Here's how the part is built. I have some questions about the finished solid (model axes, mm). Face numbers are marked on the shaded views. A direction names the side the tool comes from. Coordinates: 2 decimals unless noted, no trailing zeros. Loops run counter-clockwise (first coordinate to the right, second up) from the corner with the lowest first, then second, coordinate; pieces in that order, holes last.
```python
from build123d import *

# Parameters (mm, degrees)
EXTRUDE_2_DEPTH          = 32.5
CUT_EXTRUDE_1_DEPTH      = 64.947243881
CUT_EXTRUDE_1_DEPTH_BACK = 64.947243881
SKETCH_2_W               = 30
SKETCH_2_H               = 18
SKETCH_3_R               = 20
EXTRUDE_3_DEPTH          = 30
SKETCH_4_W               = 15
SKETCH_4_H               = 65
CUT_EXTRUDE_2_DEPTH      = 20


with BuildPart() as part:
    # Эскиз1 → Бобышка-Вытянуть2 (new, symmetric)
    with BuildSketch(Plane.XY):
        Polygon((-30, 27), (-48, -12), (-48, -27), (48, -27), (48, -12), (30, 27), align=None)
    extrude(amount=EXTRUDE_2_DEPTH, both=True)

    # Эскиз2 → Вырез-Вытянуть1 (cut, two sides: drawn at the far end of the back side and taken through both)
    with BuildSketch(Plane(origin=(0, 0, 0), x_dir=(0, 0, -1), z_dir=(1, 0, 0)).offset(-CUT_EXTRUDE_1_DEPTH_BACK)):
        with Locations((0, 7)):
            Rectangle(SKETCH_2_W, SKETCH_2_H)
    extrude(amount=CUT_EXTRUDE_1_DEPTH + CUT_EXTRUDE_1_DEPTH_BACK, mode=Mode.SUBTRACT)

    # Эскиз3 → Бобышка-Вытянуть3 (add)
    with BuildSketch(Plane(origin=(0, 27, 0), x_dir=(1, 0, 0), z_dir=(0, 1, 0))):
        with Locations(Location((0, 0, 0), (0, 0, 90))):
            Circle(SKETCH_3_R)
    extrude(amount=EXTRUDE_3_DEPTH)

    # Эскиз4 → Вырез-Вытянуть2 (cut)
    with BuildSketch(Plane(origin=(0, 57, 0), x_dir=(1, 0, 0), z_dir=(0, 1, 0))):
        Rectangle(SKETCH_4_W, SKETCH_4_H)
    extrude(amount=-CUT_EXTRUDE_2_DEPTH, mode=Mode.SUBTRACT)


solid = part.part
```
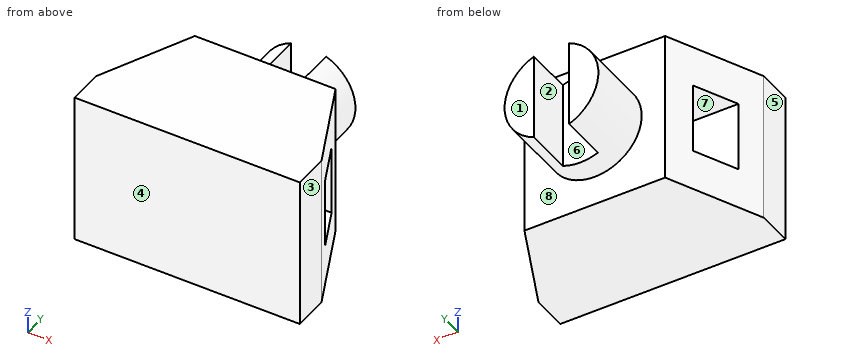
1. For pin 1 (8 mm diameter, centred on y = 0, z = 4, fed in from -X); pin 2 (6 mm diameter, centred on y = 42.5, z = -4.5, fed in from -X); pin 3 (6 mm diameter, centred on y = 43, z = 4.5, fed in from +X), each with a flat end and sliding along its axis, tell me the tip position at first contact or that it passes through.
2. I want a section at D-D (z = 27). Please give me the cut outline in (x, y).
3. I want a section at C-C (y = 50.5). Please give me the cut outline in (x, z).
4. I want a section at A-A (x = 23). Please give me the cut outline in (y, z).
5. On a 3-axis mill with a long thin cutter (end or side, diameter ignored), from which of +Z, -Z, +X, -X, +Y, -Y can I reach the whole of each face in a straight line? I mean the marked faces 4, 5, 6, 7 and 8. Say none if no direction works.
6. I need wall thicknesses on line 1 along Y through (x, z) = (12, -5); line 2 along Y through (x, z) = (-39, -4.5); line 3 along Y through (x, z) = (4.5, -15.5). Which ranges of each line are inside material? Lowest first, please.
7. I want a section at B-B (z = 0). Please give me the cut outline in (x, y), then the cut area to 3 significant figures.
8. We'd pull the mould along X, two halves only. Please class the marked faces 1, 2 and 3: +X half, -X half, draft (parallel to the pull), parting line (faces both ways), or undercut.
Response values:
1. pin 1: stops at x = -44.31
1. pin 2: stops at x = -19.94
1. pin 3: stops at x = 19.94
2. outline: (-48, -27) - (48, -27) - (48, -12) - (30, 27) - (-30, 27) - (-48, -12) - close
3. outline: (-7.5, -18.54) - (-7.5, 18.54) arc R20 ccw to start; (7.5, -18.54) arc R20 ccw to (7.5, 18.54) - close
4. outline: (-27, -32.5) - (27, -32.5) - (27, 32.5) - (-27, 32.5) - close; hole (-2, -15) - (16, -15) - (16, 15) - (-2, 15) - close
5. face 4: +Z, -Z, +X, -X, -Y
5. face 5: +Z, -Z, -X, +Y, -Y
5. face 6: +Z, -Z, +Y
5. face 7: +X, -X
5. face 8: +Y
6. line 1: y = -27 to -2, 16 to 57
6. line 2: y = -27 to -2
6. line 3: y = -27 to 37
7. outline: (-48, -27) - (48, -27) - (48, -12) - (43.38, -2) - (-43.38, -2) - (-48, -12) - close; (-35.08, 16) - (35.08, 16) - (30, 27) - (20, 27) - (20, 57) - (7.5, 57) - (7.5, 37) - (-7.5, 37) - (-7.5, 57) - (-20, 57) - (-20, 27) - (-30, 27) - close
7. area: 3,970 mm2
8. face 1: draft
8. face 2: undercut
8. face 3: +X half
